```python
from build123d import *

# Parameters (mm, degrees)
F0_R     = 5
F1_DEPTH = 7.5
F2_R     = 30
F3_DEPTH = 15
F4_SIZE  = 2.5
F6_DEPTH = 25


with BuildPart() as f1:
    # F0 (on Top) → F1 (new body, symmetric)
    with BuildSketch(Plane.XY):
        with BuildLine():
            Line((-11.2727608123, 3.5869382136), (-8.1831376229, 1.0464208357))
            ThreePointArc((-8.1831376229, 1.0464208357), (-8.249771992, 0), (-8.1831376229, -1.0464208357))
            Line((-8.1831376229, -1.0464208357), (-11.2727608123, -3.5869382136))
            Line((-11.2727608123, -3.5869382136), (-10.5073939476, -5.4346972786))
            Line((-10.5073939476, -5.4346972786), (-6.5262833734, -5.0464208357))
            ThreePointArc((-6.5262833734, -5.0464208357), (-5.8334697188, -5.8334697188), (-5.0464208357, -6.5262833734))
            Line((-5.0464208357, -6.5262833734), (-5.4346972786, -10.5073939476))
            Line((-5.4346972786, -10.5073939476), (-3.5869382136, -11.2727608123))
            Line((-3.5869382136, -11.2727608123), (-1.0464208357, -8.1831376229))
            ThreePointArc((-1.0464208357, -8.1831376229), (0, -8.249771992), (1.0464208357, -8.1831376229))
            Line((1.0464208357, -8.1831376229), (3.5869382136, -11.2727608123))
            Line((3.5869382136, -11.2727608123), (5.4346972786, -10.5073939476))
            Line((5.4346972786, -10.5073939476), (5.0464208357, -6.5262833734))
            ThreePointArc((5.0464208357, -6.5262833734), (5.8334697188, -5.8334697188), (6.5262833734, -5.0464208357))
            Line((6.5262833734, -5.0464208357), (10.5073939476, -5.4346972786))
            Line((10.5073939476, -5.4346972786), (11.2727608123, -3.5869382136))
            Line((11.2727608123, -3.5869382136), (8.1831376229, -1.0464208357))
            ThreePointArc((8.1831376229, -1.0464208357), (8.249771992, 0), (8.1831376229, 1.0464208357))
            Line((8.1831376229, 1.0464208357), (11.2727608123, 3.5869382136))
            Line((11.2727608123, 3.5869382136), (10.5073939476, 5.4346972786))
            Line((10.5073939476, 5.4346972786), (6.5262833734, 5.0464208357))
            ThreePointArc((6.5262833734, 5.0464208357), (5.8334697188, 5.8334697188), (5.0464208357, 6.5262833734))
            Line((5.0464208357, 6.5262833734), (5.4346972786, 10.5073939476))
            Line((5.4346972786, 10.5073939476), (3.5869382136, 11.2727608123))
            Line((3.5869382136, 11.2727608123), (1.0464208357, 8.1831376229))
            ThreePointArc((1.0464208357, 8.1831376229), (0, 8.249771992), (-1.0464208357, 8.1831376229))
            Line((-1.0464208357, 8.1831376229), (-3.5869382136, 11.2727608123))
            Line((-3.5869382136, 11.2727608123), (-5.4346972786, 10.5073939476))
            Line((-5.4346972786, 10.5073939476), (-5.0464208357, 6.5262833734))
            ThreePointArc((-5.0464208357, 6.5262833734), (-5.8334697188, 5.8334697188), (-6.5262833734, 5.0464208357))
            Line((-6.5262833734, 5.0464208357), (-10.5073939476, 5.4346972786))
            Line((-10.5073939476, 5.4346972786), (-11.2727608123, 3.5869382136))
        make_face()
        Circle(F0_R, mode=Mode.SUBTRACT)
    extrude(amount=F1_DEPTH, both=True)

    # F2 (on face) → F3 (join)
    with BuildSketch(Plane.XY.offset(7.5)):
        Circle(F2_R)
    extrude(amount=F3_DEPTH)

    # F4
    f4_edges = [f1.edges().sort_by_distance(p)[0] for p in [
        (-30, 0, 22.5),
        (-30, 0, 7.5),
    ]]
    chamfer(f4_edges, length=F4_SIZE)

    # F5 (on face) → F6 (cut)
    with BuildSketch(Plane.XY.offset(22.5)):
        with BuildLine():
            Line((-1, 24.9818121673), (1, 24.9818121673))
            Line((1, 24.9818121673), (1, 27.4818121673))
            ThreePointArc((1, 27.4818121673), (0, 27.5), (-1, 27.4818121673))
            Line((-1, 27.4818121673), (-1, 24.9818121673))
        make_face()
        with BuildLine():
            ThreePointArc((-7.5412904796, 26.4457735357), (-8.4979673453, 26.1540541981), (-9.4434035122, 25.827739547))
            Line((-9.4434035122, 25.827739547), (-8.6708610263, 23.4500982562))
            Line((-8.6708610263, 23.4500982562), (-6.7687479937, 24.068132245))
            Line((-6.7687479937, 24.068132245), (-7.5412904796, 26.4457735357))
        make_face()
        with BuildLine():
            ThreePointArc((-15.3443869038, 22.8210383319), (-16.164094438, 22.2479673453), (-16.9624208926, 21.6454678273))
            Line((-16.9624208926, 21.6454678273), (-15.4929577619, 19.6229253414))
            Line((-15.4929577619, 19.6229253414), (-13.8749237731, 20.7984958459))
            Line((-13.8749237731, 20.7984958459), (-15.3443869038, 22.8210383319))
        make_face()
        with BuildLine():
            ThreePointArc((-21.6454678273, 16.9624208926), (-22.2479673453, 16.164094438), (-22.8210383319, 15.3443869038))
            Line((-22.8210383319, 15.3443869038), (-20.7984958459, 13.8749237731))
            Line((-20.7984958459, 13.8749237731), (-19.6229253414, 15.4929577619))
            Line((-19.6229253414, 15.4929577619), (-21.6454678273, 16.9624208926))
        make_face()
        with BuildLine():
            ThreePointArc((-25.827739547, 9.4434035122), (-26.1540541981, 8.4979673453), (-26.4457735357, 7.5412904796))
            Line((-26.4457735357, 7.5412904796), (-24.068132245, 6.7687479937))
            Line((-24.068132245, 6.7687479937), (-23.4500982562, 8.6708610263))
            Line((-23.4500982562, 8.6708610263), (-25.827739547, 9.4434035122))
        make_face()
        with BuildLine():
            ThreePointArc((-27.4818121673, 1), (-27.5, 0), (-27.4818121673, -1))
            Line((-27.4818121673, -1), (-24.9818121673, -1))
            Line((-24.9818121673, -1), (-24.9818121673, 1))
            Line((-24.9818121673, 1), (-27.4818121673, 1))
        make_face()
        with BuildLine():
            ThreePointArc((-26.4457735357, -7.5412904796), (-26.1540541981, -8.4979673453), (-25.827739547, -9.4434035122))
            Line((-25.827739547, -9.4434035122), (-23.4500982562, -8.6708610263))
            Line((-23.4500982562, -8.6708610263), (-24.068132245, -6.7687479937))
            Line((-24.068132245, -6.7687479937), (-26.4457735357, -7.5412904796))
        make_face()
        with BuildLine():
            ThreePointArc((-22.8210383319, -15.3443869038), (-22.2479673453, -16.164094438), (-21.6454678273, -16.9624208926))
            Line((-21.6454678273, -16.9624208926), (-19.6229253414, -15.4929577619))
            Line((-19.6229253414, -15.4929577619), (-20.7984958459, -13.8749237731))
            Line((-20.7984958459, -13.8749237731), (-22.8210383319, -15.3443869038))
        make_face()
        with BuildLine():
            ThreePointArc((-16.9624208926, -21.6454678273), (-16.164094438, -22.2479673453), (-15.3443869038, -22.8210383319))
            Line((-15.3443869038, -22.8210383319), (-13.8749237731, -20.7984958459))
            Line((-13.8749237731, -20.7984958459), (-15.4929577619, -19.6229253414))
            Line((-15.4929577619, -19.6229253414), (-16.9624208926, -21.6454678273))
        make_face()
        with BuildLine():
            ThreePointArc((-9.4434035122, -25.827739547), (-8.4979673453, -26.1540541981), (-7.5412904796, -26.4457735357))
            Line((-7.5412904796, -26.4457735357), (-6.7687479937, -24.068132245))
            Line((-6.7687479937, -24.068132245), (-8.6708610263, -23.4500982562))
            Line((-8.6708610263, -23.4500982562), (-9.4434035122, -25.827739547))
        make_face()
        with BuildLine():
            ThreePointArc((-1, -27.4818121673), (0, -27.5), (1, -27.4818121673))
            Line((1, -27.4818121673), (1, -24.9818121673))
            Line((1, -24.9818121673), (-1, -24.9818121673))
            Line((-1, -24.9818121673), (-1, -27.4818121673))
        make_face()
        with BuildLine():
            ThreePointArc((7.5412904796, -26.4457735357), (8.4979673453, -26.1540541981), (9.4434035122, -25.827739547))
            Line((9.4434035122, -25.827739547), (8.6708610263, -23.4500982562))
            Line((8.6708610263, -23.4500982562), (6.7687479937, -24.068132245))
            Line((6.7687479937, -24.068132245), (7.5412904796, -26.4457735357))
        make_face()
        with BuildLine():
            ThreePointArc((15.3443869038, -22.8210383319), (16.164094438, -22.2479673453), (16.9624208926, -21.6454678273))
            Line((16.9624208926, -21.6454678273), (15.4929577619, -19.6229253414))
            Line((15.4929577619, -19.6229253414), (13.8749237731, -20.7984958459))
            Line((13.8749237731, -20.7984958459), (15.3443869038, -22.8210383319))
        make_face()
        with BuildLine():
            ThreePointArc((21.6454678273, -16.9624208926), (22.2479673453, -16.164094438), (22.8210383319, -15.3443869038))
            Line((22.8210383319, -15.3443869038), (20.7984958459, -13.8749237731))
            Line((20.7984958459, -13.8749237731), (19.6229253414, -15.4929577619))
            Line((19.6229253414, -15.4929577619), (21.6454678273, -16.9624208926))
        make_face()
        with BuildLine():
            ThreePointArc((25.827739547, -9.4434035122), (26.1540541981, -8.4979673453), (26.4457735357, -7.5412904796))
            Line((26.4457735357, -7.5412904796), (24.068132245, -6.7687479937))
            Line((24.068132245, -6.7687479937), (23.4500982562, -8.6708610263))
            Line((23.4500982562, -8.6708610263), (25.827739547, -9.4434035122))
        make_face()
        with BuildLine():
            ThreePointArc((27.4818121673, -1), (27.5, 0), (27.4818121673, 1))
            Line((27.4818121673, 1), (24.9818121673, 1))
            Line((24.9818121673, 1), (24.9818121673, -1))
            Line((24.9818121673, -1), (27.4818121673, -1))
        make_face()
        with BuildLine():
            ThreePointArc((26.4457735357, 7.5412904796), (26.1540541981, 8.4979673453), (25.827739547, 9.4434035122))
            Line((25.827739547, 9.4434035122), (23.4500982562, 8.6708610263))
            Line((23.4500982562, 8.6708610263), (24.068132245, 6.7687479937))
            Line((24.068132245, 6.7687479937), (26.4457735357, 7.5412904796))
        make_face()
        with BuildLine():
            ThreePointArc((22.8210383319, 15.3443869038), (22.2479673453, 16.164094438), (21.6454678273, 16.9624208926))
            Line((21.6454678273, 16.9624208926), (19.6229253414, 15.4929577619))
            Line((19.6229253414, 15.4929577619), (20.7984958459, 13.8749237731))
            Line((20.7984958459, 13.8749237731), (22.8210383319, 15.3443869038))
        make_face()
        with BuildLine():
            ThreePointArc((16.9624208926, 21.6454678273), (16.164094438, 22.2479673453), (15.3443869038, 22.8210383319))
            Line((15.3443869038, 22.8210383319), (13.8749237731, 20.7984958459))
            Line((13.8749237731, 20.7984958459), (15.4929577619, 19.6229253414))
            Line((15.4929577619, 19.6229253414), (16.9624208926, 21.6454678273))
        make_face()
        with BuildLine():
            ThreePointArc((9.4434035122, 25.827739547), (8.4979673453, 26.1540541981), (7.5412904796, 26.4457735357))
            Line((7.5412904796, 26.4457735357), (6.7687479937, 24.068132245))
            Line((6.7687479937, 24.068132245), (8.6708610263, 23.4500982562))
            Line((8.6708610263, 23.4500982562), (9.4434035122, 25.827739547))
        make_face()
    extrude(amount=-F6_DEPTH, mode=Mode.SUBTRACT)


solid = f1.part
```
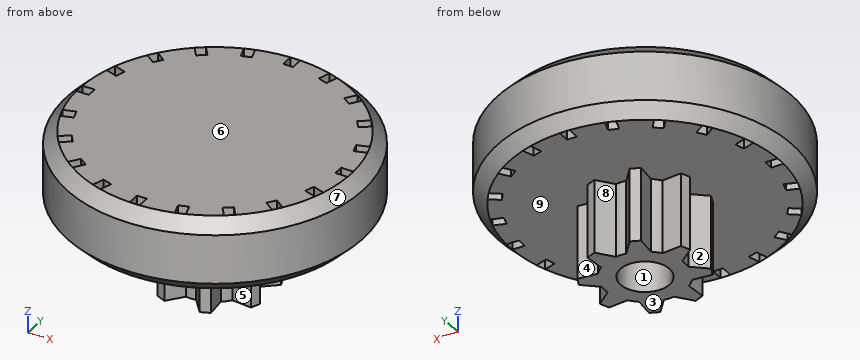
Read the model definition and answer for the solid it produces. Units are mm, in the model's axes. Face numbers are marked on the shaded views. A direction names the side the tool comes from. Round coordinates to 2 decimals unless told otherwise and drop trailing zeros. Loops run counter-clockwise (first coordinate to the right, second up) from the corner with the lowest first, then second, coordinate; pieces in that order, holes last. Notation, with made-up numbers: (35, 7.5) -> (42, 7.5) arc R31 cw to (42, 41.5) -> close; hole circle Ø11 at (87, 28). An arc over 180 degrees is marked (long way). One line per item, written item: value.
1) Consider L1, parallel to Y at x = 0, z = -0.75; L2, parallel to X at y = 8, z = 11.5; L3, parallel to X at y = -22.5, z = 15. Determine where each line is inside the solid, lowest interval first. Write a range as [from, to].
Answer list:
L1: y = [-8.25, -5], [5, 8.25]
L2: x = [-28.91, -26.31], [-23.67, 23.67], [26.31, 28.91]
L3: x = [-19.84, -15.81], [-15.11, 15.11], [15.81, 19.84]
2) Flat-ended cylindrical pins translate along their axes: P1, Ø3, axis at x = 26, z = 17.5, coming from the -Y side; P2, Ø0.8, axis at y = 26.5, z = 14.5, coming from the -X side; P3, Ø10, axis at y = -13, z = 15.5, coming from the +X side. Find the tip coordinate at first contact, or state that the pin passes through.
Answer list:
P1: stops at y = -17.31
P2: stops at x = -14.79
P3: stops at x = 28.91
3) A cutting plane is placed at D-D (z = 12.75). Give the number of separate pieces and of enclosed holes in the cut face, and give its area (3 significant figures).
Answer list:
separate pieces: 1
enclosed holes: 20
area: 2,730 mm²
4) A cutting plane is placed at B-B (y = 0). Determine the outline of the cut face in (x, z), and give its area (3 significant figures).
Answer list:
outline: (-30, 10) -> (-27.5, 7.5) -> (-27.5, 22.5) -> (-30, 20) -> close; (-24.98, 7.5) -> (-8.25, 7.5) -> (-8.25, -7.5) -> (-5, -7.5) -> (-5, 7.5) -> (5, 7.5) -> (5, -7.5) -> (8.25, -7.5) -> (8.25, 7.5) -> (24.98, 7.5) -> (24.98, 22.5) -> (-24.98, 22.5) -> close; (27.5, 7.5) -> (30, 10) -> (30, 20) -> (27.5, 22.5) -> close
area: 909 mm²
5) For the marked faces 5, 6, 7, 8 and 9, determine the directions among +Z, -Z, +X, -X, +Y, -Y from which every point of the face is accessible in a straight line to the end or side of a thin tool.
Answer list:
face 5: -Z, -Y
face 6: +Z, +X, -X, +Y, -Y
face 7: +Z
face 8: -Z, +Y
face 9: -Z
6) The mould has two halves that part along X. Classify the marked faces 1, 2, 3 and 4: pulls with the +X half, pulls with the -X half, needs draft (parallel to the pull), parting line crosses it, or undercut.
Answer list:
face 1: undercut
face 2: pulls with the -X half
face 3: needs draft
face 4: undercut
